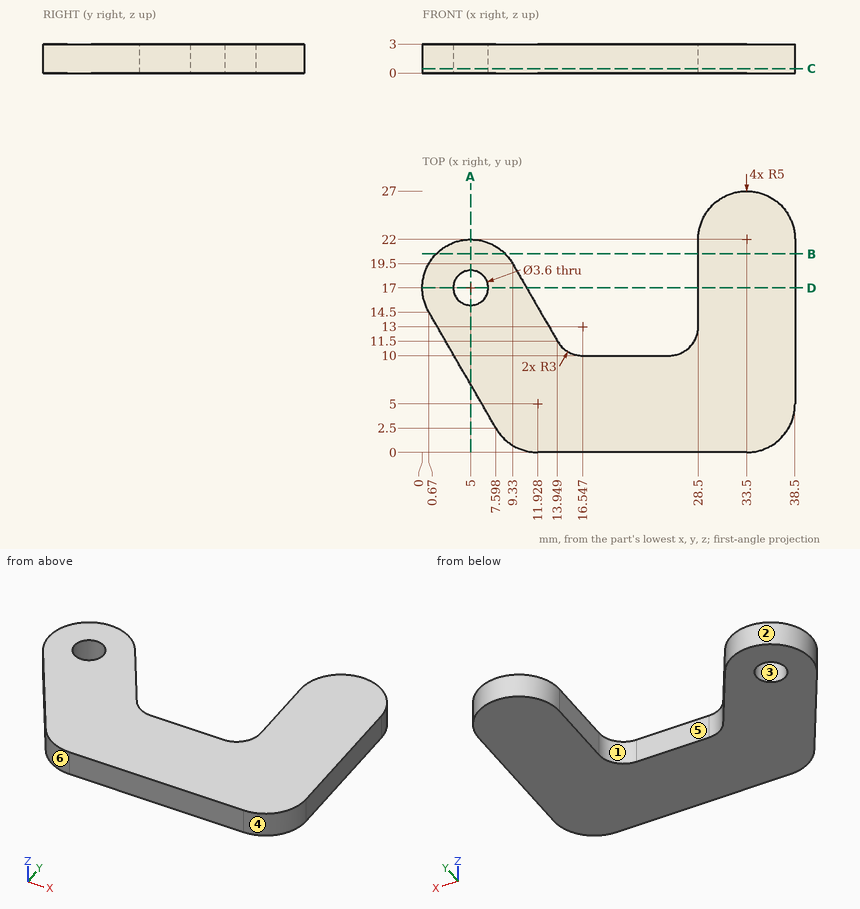
Can you work these out from the drawing? Everything is in mm from the part's minimum corner. A direction names the side the tool comes from. Give positions to 0.01 mm unless a question says otherwise; leave off trailing zeros. Order: outer loops, then holes, each group sorted by start corner. A loop starts at its lowest first (then second) coordinate and runs counter-clockwise, first axis right, second up. Notation, with made-up numbers: (35, 5.5) -> (59, 5.5) arc R27 cw to (59, 31.5) -> close; hole circle Ø8 at (87.5, 87.5). An arc over 180 degrees is marked (long way). Return JSON: item names as keys, results as strings.
1. Thinking about a two-plate mould opening in X: for the marked faces 3, 4, 5 and 6, which applies, pulls with the +X half, pulls with the -X half, needs draft (parallel to the pull), parting line crosses it, or undercut?
Answer list:
{"face 3": "undercut", "face 4": "pulls with the +X half", "face 5": "undercut", "face 6": "pulls with the -X half"}
2. Imagine slicing it at D-D on y = 17. List the corners of the cut face in (x, z) for me.
Answer list:
{"outline": "(0, 0) -> (3.2, 0) -> (3.2, 3) -> (0, 3) -> close; (6.8, 0) -> (10.77, 0) -> (10.77, 3) -> (6.8, 3) -> close; (28.5, 0) -> (38.5, 0) -> (38.5, 3) -> (28.5, 3) -> close"}
3. Imagine slicing it at B-B on y = 20.5. List the corners of the cut face in (x, z) for me, then the cut area to 3 significant figures.
Answer list:
{"outline": "(1.43, 0) -> (8.57, 0) -> (8.57, 3) -> (1.43, 3) -> close; (28.5, 0) -> (38.5, 0) -> (38.5, 3) -> (28.5, 3) -> close", "area": "51.4 mm2"}
4. Imagine slicing it at A-A on x = 5. List the corners of the cut face in (y, z) for me, then the cut area to 3 significant figures.
Answer list:
{"outline": "(7, 0) -> (15.2, 0) -> (15.2, 3) -> (7, 3) -> close; (18.8, 0) -> (22, 0) -> (22, 3) -> (18.8, 3) -> close", "area": "34.2 mm2"}
5. On a 3-axis mill with a long thin cutter (end or side, diameter ignored), from which of +Z, -Z, +X, -X, +Y, -Y can I reach the whole of each face in a straight line? I mean the marked faces 1 and 2. Say none if no direction works.
Answer list:
{"face 1": "+Z, -Z, +Y", "face 2": "+Z, -Z"}
6. I need wall thicknesses on line 1 (X direction, y = 13, z = 0.55); line 2 (X direction, y = 17.5, z = 1.2) (1 decimal); line 3 (X direction, y = 12, z = 0.3). Which ranges of each line are inside material? Lowest first, please. Write a range as from..to.
Answer list:
{"line 1": "x = 1.54..13.08, 28.5..38.5", "line 2": "x = 0..3.3, 6.7..10.5, 28.5..38.5", "line 3": "x = 2.11..13.66, 28.33..38.5"}
7. Imagine slicing it at C-C on z = 0.45. List the corners of the cut face in (x, y) for me.
Answer list:
{"outline": "(0.67, 14.5) -> (7.6, 2.5) arc R5 ccw to (11.93, 0) -> (33.5, 0) arc R5 ccw to (38.5, 5) -> (38.5, 22) arc R5 ccw to (28.5, 22) -> (28.5, 13) arc R3 cw to (25.5, 10) -> (16.55, 10) arc R3 cw to (13.95, 11.5) -> (9.33, 19.5) arc R5 ccw to start; hole circle Ø3.6 at (5, 17)"}
